Verification items for the finished model (mm, model axes). A direction names the side the tool comes from. Give positions to 0.01 mm unless a question says otherwise; leave off trailing zeros. Write each loop counter-clockwise with the first axis right and the second up, starting at its lowest first coordinate (ties: lowest second). Pieces come first, ordered by that corner, then holes.
from build123d import *

# Parameters (mm, degrees)
SKETCH1_R                              = 10
BOSS_EXTRUDE1_DEPTH                    = 22
SKETCH6_R                              = 11
BOSS_EXTRUDE2_DEPTH                    = 11
F_8_0MM_DOWEL_HOLE1_D                  = 8
F_8_0MM_DOWEL_HOLE1_CSINK_D            = 8.05
F_8_0MM_DOWEL_HOLE1_CSINK_ANGLE        = 90
SKETCH9_R                              = 15.792919945
CUT_EXTRUDE1_DEPTH                     = 3
SKETCH8_R                              = 3
BOSS_EXTRUDE3_DEPTH                    = 21
SKETCH10_W                             = 4
SKETCH10_H                             = 22
BOSS_EXTRUDE4_DEPTH                    = 19
BOSS_EXTRUDE5_START                    = -3
BOSS_EXTRUDE5_DEPTH                    = 3
SKETCH12_W                             = 26
SKETCH12_H                             = 28
SKETCH12_W_2                           = 20
SKETCH12_H_2                           = 22
CUT_EXTRUDE2_DEPTH                     = 47.957427527
TAP_DRILL_FOR_M3_HELICOIL1_D           = 3.15
TAP_DRILL_FOR_M3_HELICOIL1_DEPTH       = 6
TAP_DRILL_FOR_M3_HELICOIL1_CSINK_D     = 3.2
TAP_DRILL_FOR_M3_HELICOIL1_CSINK_ANGLE = 90
TAP_DRILL_FOR_M3_HELICOIL1_TIP         = 0.946355475


with BuildPart() as part:
    # Sketch1 → Boss-Extrude1 (new body)
    with BuildSketch(Plane.XY):
        Circle(SKETCH1_R)
    extrude(amount=BOSS_EXTRUDE1_DEPTH)

    # Sketch6 → Boss-Extrude2 (add, symmetric)
    with BuildSketch(Plane(origin=(0, 0, 0), x_dir=(1, 0, 0), z_dir=(0, 1, 0))):
        with Locations(Location((0, -11, 0), (0, 0, 270))):
            Circle(SKETCH6_R)
    extrude(amount=BOSS_EXTRUDE2_DEPTH, both=True)

    # Ø8.0mm Dowel Hole1 (through all)
    with Locations(Plane.XY.offset(22)):
        with Locations((0, 0)):
            CounterSinkHole(F_8_0MM_DOWEL_HOLE1_D / 2, F_8_0MM_DOWEL_HOLE1_CSINK_D / 2, counter_sink_angle=F_8_0MM_DOWEL_HOLE1_CSINK_ANGLE)

    # Sketch9 → Cut-Extrude1 (cut)
    with BuildSketch(Plane(origin=(0, 11, 0), x_dir=(1, 0, 0), z_dir=(0, 1, 0))):
        with Locations((0, -11)):
            Circle(SKETCH9_R)
    extrude(amount=-CUT_EXTRUDE1_DEPTH, mode=Mode.SUBTRACT)

    # Sketch8 → Boss-Extrude3 (add)
    with BuildSketch(Plane(origin=(0, 8, 0), x_dir=(1, 0, 0), z_dir=(0, 1, 0))):
        with Locations(Location((0, -11, 0), (0, 0, 90))):
            Circle(SKETCH8_R)
    extrude(amount=BOSS_EXTRUDE3_DEPTH)

    # Sketch10 → Boss-Extrude4 (add)
    with BuildSketch(Plane(origin=(0, 8, 0), x_dir=(1, 0, 0), z_dir=(0, 1, 0))):
        with Locations((-8, -11)):
            Rectangle(SKETCH10_W, SKETCH10_H)
        with Locations((8, -11)):
            Rectangle(SKETCH10_W, SKETCH10_H)
    extrude(amount=-BOSS_EXTRUDE4_DEPTH)

    # Sketch11 → Boss-Extrude5 (add)
    with BuildSketch(Plane.XZ.offset(11).offset(BOSS_EXTRUDE5_START)):
        with BuildLine():
            Line((0, 22), (-6, 22))
            Line((-6, 22), (-6, 20.219544457))
            ThreePointArc((-6, 20.219544457), (-3.129297922, 21.545496409), (0, 22))
        make_face()
        with BuildLine():
            Line((6, 22), (0, 22))
            ThreePointArc((0, 22), (3.129297922, 21.545496409), (6, 20.219544457))
            Line((6, 20.219544457), (6, 22))
        make_face()
        with BuildLine():
            Line((-6, 1.780455543), (-6, 0))
            Line((-6, 0), (-1.12e-07, 0))
            ThreePointArc((-1.12e-07, 0), (-3.129297976, 0.454503607), (-6, 1.780455543))
        make_face()
        with BuildLine():
            ThreePointArc((6, 1.780455543), (3.129297868, 0.454503575), (-1.12e-07, 0))
            Line((-1.12e-07, 0), (6, 0))
            Line((6, 0), (6, 1.780455543))
        make_face()
    extrude(amount=BOSS_EXTRUDE5_DEPTH)

    # Sketch12 → Cut-Extrude2 (cut, through all)
    with BuildSketch(Plane.XZ.offset(11)):
        with Locations((0, 11)):
            Rectangle(SKETCH12_W, SKETCH12_H)
        with Locations((0, 11)):
            Rectangle(SKETCH12_W_2, SKETCH12_H_2, mode=Mode.SUBTRACT)
    extrude(amount=-CUT_EXTRUDE2_DEPTH, mode=Mode.SUBTRACT)

    # Tap Drill for M3 Helicoil1
    with Locations(Plane(origin=(0, 29, 0), x_dir=(1, 0, 0), z_dir=(0, 1, 0))):
        with Locations((0, -11)):
            CounterSinkHole(TAP_DRILL_FOR_M3_HELICOIL1_D / 2, TAP_DRILL_FOR_M3_HELICOIL1_CSINK_D / 2, depth=TAP_DRILL_FOR_M3_HELICOIL1_DEPTH, counter_sink_angle=TAP_DRILL_FOR_M3_HELICOIL1_CSINK_ANGLE)
            with Locations((0, 0, -(TAP_DRILL_FOR_M3_HELICOIL1_DEPTH + TAP_DRILL_FOR_M3_HELICOIL1_TIP / 2))):  # 118° drill point
                Cone(0, TAP_DRILL_FOR_M3_HELICOIL1_D / 2, TAP_DRILL_FOR_M3_HELICOIL1_TIP, mode=Mode.SUBTRACT)


solid = part.part
Item 1: Scan lines: line 1 along X through (y, z) = (0, 10); line 2 along X through (y, z) = (26.95, 11) (3 decimals); line 3 along Y through (x, z) = (0, 10.25). Record each from-to range of solid material in increasing order.
Answer key:
line 1: x = -10 to -4, 4 to 10
line 2: x = -3 to -1.575, 1.575 to 3
line 3: y = -11 to -4, 4 to 22.5
Item 2: Sectioned sample at D-D on y = 24. Record the cut outline in (x, z) (3 decimals).
Answer key:
outline: circle Ø6 at (0, 11); hole circle Ø3.15 at (0, 11)
Item 3: Sectioned sample at A-A on y = 0. Record the cut outline in (x, z) (3 decimals), then the cut area to 3 significant figures.
Answer key:
outline: (-10, 0) - (-4, 0) - (-4, 21.975) - (-4.025, 22) - (-10, 22) - close; (4, 0) - (10, 0) - (10, 22) - (4.025, 22) - (4, 21.975) - close
area: 264 mm2
Item 4: Release check for a two-part mould opening along Y. For faces 1 (the face through (0.341, 25.946, 12.538)), 2 (the face through (0.126, 22.218, 11.243)), 3 (the face through (0.867, -3.905, 10.834)) record: released by +Y, released by -Y, zero draft, split by the parting line, or undercut.
Answer key:
face 1: zero draft
face 2: released by +Y
face 3: undercut
Item 5: Sectioned sample at B-B on z = 15.5. Record the cut outline in (x, y).
Answer key:
outline: (-10, -11) - (10, -11) - (10, 8) - (-10, 8) - close; hole circle Ø8 at (0, 0)
Item 6: Set-up check for faces 4 (the face through (0, 18, 14)), 5 (the face through (0, -11, 11)): record each of +Z, -Z, +X, -X, +Y, -Y from which the full face is reachable in a straight line by a thin tool's end or side.
Answer key:
face 4: +Y
face 5: +Z, -Z, +X, -X, -Y
Item 7: Sectioned sample at C-C on x = -8. Record the cut outline in (y, z).
Answer key:
outline: (-11, 0) - (8, 0) - (8, 22) - (-11, 22) - close
Item 8: Depth check by flat-ended pin: pin 1 (6 mm diameter, centred on x = -7, y = 24, fed in from +Z); pin 2 (6 mm diameter, centred on x = 2, y = 16, fed in from +Z). Enter the tip coordinate at first touch or a pass-through.
Answer key:
pin 1: passes through
pin 2: stops at z = 14
